Model file for the job. Use its own axes, mm. Coordinates: 2 decimals unless noted, no trailing zeros. Order: outer loops, then holes, each group sorted by start corner. A loop starts at its lowest first (then second) coordinate and runs counter-clockwise, first axis right, second up. Notation, with made-up numbers: (82.25, 27.25) -> (132.25, 27.25) arc R15 ccw to (132.25, 33.25) -> close; hole circle Ø9 at (81, 75.5). An arc over 180 degrees is marked (long way). Write item = value, one per line. Start each with the question number.
Q1. Flat gauge pin, fed straight in: pin 1 (5 mm diameter, centred on x = 149, y = 7.5, fed in from +Z). Where does the tip first touch, or does it go through?
Q2. Cut at A-A, the plane z = -1054.5. List the corners of the cut face in (x, y), plus the area to 3 significant figures.
Q3. Wall check: line 1 (Z direction, x = -92, y = 6); line 2 (Z direction, x = -185, y = 4). Give the ranges that are in metal, low to high. Write a range as from..to.
Q4. Cut at D-D, the plane x = 6. List the corners of the cut face in (y, z).
Q5. Cut at C-C, the plane z = -1028. List the corners of the cut face in (x, y), plus the area to 3 significant figures.
Q6. Cut at B-B, the plane y = 1.5. List the corners of the cut face in (x, z).
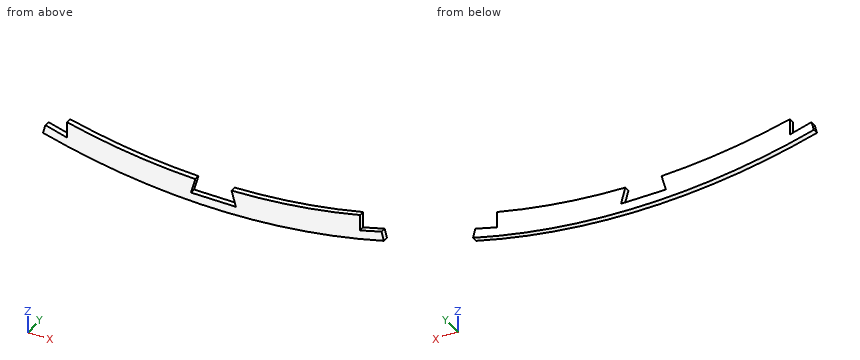
from build123d import *

# Parameters (mm, degrees)
BOSS_EXTRUDE1_DEPTH = 9


with BuildPart() as part:
    # Sketch1 → Boss-Extrude1 (new body)
    with BuildSketch(Plane(origin=(0, 0, 0), x_dir=(1, 0, 0), z_dir=(0, 1, 0))):
        with BuildLine():
            Line((-280.818663936, 1048.029521524), (-276.93637826, 1033.540634129))
            Line((-276.93637826, 1033.540634129), (-241.197122687, 1043.116938798))
            Line((-241.197122687, 1043.116938798), (-241.488127343, 1017.157059825))
            Line((-241.488127343, 1017.157059825), (-241.493100981, 1016.713372676))
            ThreePointArc((-241.493100981, 1016.713372676), (-136.39987087, 1036.059880136), (-29.880361151, 1044.572718396))
            Line((-29.880361151, 1044.572718396), (-30, 1045))
            Line((-30, 1045), (-37, 1070))
            Line((-37, 1070), (37, 1070))
            Line((37, 1070), (30, 1045))
            Line((30, 1045), (29.880361151, 1044.572718396))
            ThreePointArc((29.880361151, 1044.572718396), (136.39987087, 1036.059880136), (241.493100981, 1016.713372676))
            Line((241.493100981, 1016.713372676), (241.488127343, 1017.157059825))
            Line((241.488127343, 1017.157059825), (241.197122687, 1043.116938798))
            Line((241.197122687, 1043.116938798), (276.93637826, 1033.540634129))
            Line((276.93637826, 1033.540634129), (280.818663936, 1048.029521524))
            ThreePointArc((280.818663936, 1048.029521524), (0, 1085), (-280.818663936, 1048.029521524))
        make_face()
    extrude(amount=BOSS_EXTRUDE1_DEPTH)


solid = part.part
Here are the results:
q1.pin_1 = -1033.96
q2.outline = (-255.45, 0) -> (-32.66, 0) -> (-32.66, 9) -> (-255.45, 9) -> close; (32.66, 0) -> (255.45, 0) -> (255.45, 9) -> (32.66, 9) -> close
q2.area = 4,010 mm²
q3.line_1 = -1081.09..-1040.94
q3.line_2 = -1069.11..-1028.49
q4.outline = (0, -1084.98) -> (9, -1084.98) -> (9, -1070) -> (0, -1070) -> close
q5.outline = (-241.37, 0) -> (-187.73, 0) -> (-187.73, 9) -> (-241.37, 9) -> close; (187.73, 0) -> (241.37, 0) -> (241.37, 9) -> (187.73, 9) -> close
q5.area = 966 mm²
q6.outline = (-280.82, -1048.03) arc R1085 ccw to (280.82, -1048.03) -> (276.94, -1033.54) -> (241.2, -1043.12) -> (241.49, -1016.71) arc R1045 cw to (29.88, -1044.57) -> (37, -1070) -> (-37, -1070) -> (-29.88, -1044.57) arc R1045 cw to (-241.49, -1016.71) -> (-241.2, -1043.12) -> (-276.94, -1033.54) -> close
